Autodesk Inventor part; units mm, degrees
ref_plane "YZ Plane" through (0, 0, 0) normal (1, 0, 0) x (0, 1, 0)
ref_plane "XZ Plane" through (0, 0, 0) normal (0, 1, 0) x (-1, 0, 0)
ref_plane "XY Plane" through (0, 0, 0) normal (0, 0, 1) x (1, 0, 0)
sketch "Sketch1" plane through (0, 0, 0) normal (0, 0, 1) x (1, 0, 0)
  line L0 (-2, 7) -> (26, 7)
  line L1 (-13.8022, 0) -> (14.1978, 0) construction
  line L2 (26, 7) -> (26, 13)
  line L3 (26, 13) -> (24, 13)
  line L4 (24, 13) -> (24, 28)
  line L5 (0, 28) -> (0, 13)
  line L6 (0, 13) -> (-2, 13)
  line L7 (-2, 13) -> (-2, 7)
  arc A0 (2.202, 28) -> (21.798, 28) centre (12, 38) ccw
  arc A1 (2.202, 28) -> (21.798, 28) centre (12, 38) ccw
  line L8 (2.202, 28) -> (0, 28)
  line L9 (21.798, 28) -> (24, 28)
  point P0 (0, 0)
  dimension "d0" = 28
  dimension "d1" = 14
  dimension "d2" = 26
  dimension "d3" = 2
  dimension "d5" = 24
  dimension "d11" = 14
  dimension "d12" = 56
  dimension "d13" = 76
revolve "Revolution1" add sketch "Sketch1" angle 360 about axis through (-13.8022, 0, 0) along (1, 0, 0)
fillet "Fillet1" radius 2 2 edges at (24, -13, 0) (0, -13, 0)
properties part number "parte2_revolucion"
Model file for the job. Use its own axes, mm. A direction names the side the tool comes from. Coordinates: 2 decimals unless noted, no trailing zeros. Loops run counter-clockwise (first coordinate to the right, second up) from the corner with the lowest first, then second, coordinate; pieces in that order, holes last. Notation, with made-up numbers: (52.25, 45.5) - (87.25, 45.5) arc R13 ccw to (87.25, 49.5) - close; hole circle Ø3 at (16, 60). An arc over 180 degrees is marked (long way). Write item = value, one per line. Start each with the question number.
Item 1: Drop flat-ended pins along their axis: pin 1 Ø4 at (y, z) = (19.5, 20) entering from -X; pin 2 Ø4 at (x, z) = (9.5, 17.5) entering from +Y; pin 3 Ø8 at (x, y) = (13, 9) entering from -Z; pin 4 Ø18 at (y, z) = (0, 0) entering from +X. Give the stop position or say it passes through.
Item 2: Saw through at C-C, the plane x = 12.5. List the corners of the cut face in (y, z), then the cut area to 3 significant figures.
Item 3: Saw through at D-D, the plane x = 5. List the corners of the cut face in (y, z), then the cut area to 3 significant figures.
Item 4: 3-axis set-ups, long thin cutter, end or side, ignore diameter. For faces 1 (the face through (24, 12, -12)), 2 (the face through (26, 6, -6)): which of +Z, -Z, +X, -X, +Y, -Y reach the whole face in a straight line?
Item 5: Pull direction Z, two halves, no side cores. Call faces 3 (the face through (12.196, 6.466, -2.681)), 4 (the face through (1.086, 25.865, 10.724)), 5 (the face through (0, 12, -12)): +Z half, -Z half, draft (parallel to the pull), parting line (faces both ways), or undercut.
Item 6: Wall check: probe 1 along X at (y, z) = (12, 14); probe 2 along Z at (x, y) = (8.25, 0); probe 3 along Z at (x, y) = (22.25, -5.5). Give the ranges that are in metal, low to high. Write a range as [from, to].
Answers:
q1.pin_1 = 0
q1.pin_2 = 18.7
q1.pin_3 = -23.75
q1.pin_4 = 26
q2.outline = circle Ø48.02 at (0, 0); hole circle Ø14 at (0, 0)
q2.area = 1,660 mm2
q3.outline = circle Ø51.75 at (0, 0); hole circle Ø14 at (0, 0)
q3.area = 1,950 mm2
q4.face_1 = +X
q4.face_2 = +Z, -Z, +X, +Y, -Y
q5.face_3 = undercut
q5.face_4 = parting line
q5.face_5 = draft
q6.probe_1 = [0, 24]
q6.probe_2 = [-24.51, -7], [7, 24.51]
q6.probe_3 = [-27.45, -4.33], [4.33, 27.45]
